from build123d import *

# Parameters (mm, degrees)
F1_DEPTH = 20
F2_R     = 2
F4_D     = 6


with BuildPart() as f1:
    # F0 (on Front) → F1 (new body)
    with BuildSketch(Plane.XZ):
        with BuildLine():
            ThreePointArc((0, 5), (1.4644660941, 1.4644660941), (5, 0))
            Line((5, 0), (84.7101905787, 0))
            ThreePointArc((84.7101905787, 0), (87.9241286272, 1.1697777844), (89.6342293438, 4.1317591117))
            Line((89.6342293438, 4.1317591117), (94.9240387651, 34.1317591117))
            ThreePointArc((94.9240387651, 34.1317591117), (94.9809734905, 34.5642212863), (95, 35))
            ThreePointArc((95, 35), (93.5355339059, 38.5355339059), (90, 40))
            Line((90, 40), (45.9883344131, 40))
            ThreePointArc((45.9883344131, 40), (42.3019477291, 38.3779510381), (41.0073609227, 34.5642212863))
            Line((41.0073609227, 34.5642212863), (41.9809734905, 23.4357787137))
            ThreePointArc((41.9809734905, 23.4357787137), (40.6863866841, 19.6220489619), (37, 18))
            Line((37, 18), (10, 18))
            ThreePointArc((10, 18), (2.9289321881, 15.0710678119), (0, 8))
            Line((0, 8), (0, 5))
        make_face()
        with BuildLine():
            ThreePointArc((49.6427151282, 27.651377029), (50.6783845734, 30.7023608305), (53.6274939206, 32))
            Line((53.6274939206, 32), (81.6577248518, 32))
            ThreePointArc((81.6577248518, 32), (85.6358124333, 28.4181138531), (82.4893716151, 24.0874095971))
            Line((82.4893716151, 24.0874095971), (54.9708824747, 18.238174163))
            ThreePointArc((54.9708824747, 18.238174163), (51.7599445644, 18.9353371235), (50.154456919, 21.802141595))
            Line((50.154456919, 21.802141595), (49.6427151282, 27.651377029))
        make_face(mode=Mode.SUBTRACT)
    extrude(amount=F1_DEPTH)

    # F2
    f2_edges = [f1.edges().sort_by_distance(p)[0] for p in [
        (67.642609, -20, 32),
        (41.494167, -20, 29),
        (68.730127, 0, 21.162792),
        (41.494167, 0, 29),
    ]]
    fillet(f2_edges, radius=F2_R)

    # F4 (through all)
    with Locations(Plane(origin=(0, 0, 0), x_dir=(1, 0, 0), z_dir=(0, 1, 0))):
        with Locations((12, -6), (80, -6)):
            Hole(F4_D / 2)


solid = f1.part
Geometry: final body of the model. Coordinates: model frame, mm. A direction names the side the tool comes from. Round coordinates to 2 decimals unless told otherwise and drop trailing zeros. Loops run counter-clockwise (first coordinate to the right, second up) from the corner with the lowest first, then second, coordinate; pieces in that order, holes last. Notation, with made-up numbers: M -34,-10.5 L -2,-10.5 A11 ccw -2,8.5 Z; hole C -6.75,-16 d5. An arc over 180 degrees is marked long. Put each result on its own line as item: value. Start each with the question number.
(1) Section query A-A (x = 12). Return loops of the section in (y, z).
(2) Section query C-C (x = 80). State how many separate pieces and enclosed holes the cut face has, then the cut area to 3 significant figures.
(3) Section query B-B (x = 26). Return loops of the section in (y, z), then the cut area to 3 significant figures.
(4) Draft query along Z for faces 1 (the face through (44, -10, 0)), 2 (the face through (0, -10, 7)), 3 (the face through (14.21, -10.14, 3.97)), 4 (the face through (67.84, -19.4, 32.57)). Return one class per face: +Z half, -Z half, draft (parallel to the pull), parting line (faces both ways), or undercut.
(5) Set-up query: faces 5 (the face through (68.656, -19.399, 20.564)), 6 (the face through (41.487, -9.888, 29.078)), 7 (the face through (23.31, -19.4, 17.43)), 8 (the face through (42.07, -19.4, 28.97)), 9 (the face through (49.327, -0.601, 24.718)). Return all of +Z, -Z, +X, -X, +Y, -Y with unobstructed straight access to the full face (end or side cutting, diameter ignored); none if empty.
(6) Contact query for flat-ended pins moving along their axis: pin 1 Ø8 at (y, z) = (-10, 23.5) entering from -X; pin 2 Ø2 at (y, z) = (-3, 25) entering from +X; pin 3 Ø5 at (y, z) = (-17.5, 26.5) entering from +X. Output: stop coordinate, or through.
(7) Material intervals for line 1 along Z through (x, y) = (12, -12.25); line 2 along Z through (x, y) = (80, -9.25); line 3 along Z through (x, y) = (81, -18.5), sorted ascending. Write a range as [from, to].
Findings below:
1. outline: M -20,2 A2 ccw -18,0 L -2,0 A2 ccw 0,2 L 0,3 L -20,3 Z; M -20,9 L 0,9 L 0,16 A2 ccw -2,18 L -18,18 A2 ccw -20,16 Z
2. separate pieces: 3
2. enclosed holes: 0
2. area: 504 mm2
3. outline: M -20,2 A2 ccw -18,0 L -2,0 A2 ccw 0,2 L 0,16 A2 ccw -2,18 L -18,18 A2 ccw -20,16 Z
3. area: 357 mm2
4. face 1: -Z half
4. face 2: draft
4. face 3: undercut
4. face 4: undercut
5. face 5: -Y
5. face 6: -X, +Y, -Y
5. face 7: +Z, -X, -Y
5. face 8: -X, -Y
5. face 9: +Y
6. pin 1: stops at x = 40.57
6. pin 2: stops at x = 93.49
6. pin 3: stops at x = 94.02
7. line 1: z = [0, 3], [9, 18]
7. line 2: z = [0, 3], [9, 23.56], [32, 40]
7. line 3: z = [0.06, 3.17], [8.83, 23.71], [32.06, 39.94]
